```python
from build123d import *

# Parameters (mm, degrees)
F0_R          = 54.61
F0_R_2        = 51.435
F1_DEPTH      = 3.175
F2_R          = 1.27
F3_DEPTH      = 59.69
F3_DEPTH_BACK = 59.69
F4_R          = 51.435
F5_DEPTH      = 25.4
F6_R          = 1.524
F7_DEPTH      = 53.975
F7_DEPTH_BACK = 53.975


with BuildPart() as f1:
    # F0 (on Top) → F1 (new body)
    with BuildSketch(Plane.XY):
        Circle(F0_R)
        Circle(F0_R_2, mode=Mode.SUBTRACT)
    extrude(amount=F1_DEPTH)

    # F2 (on Front) → F3 (join, two sides)
    with BuildSketch(Plane.XZ) as f3_sk:
        with Locations((0, 1.5875)):
            Circle(F2_R)
    extrude(amount=F3_DEPTH)
    extrude(f3_sk.sketch, amount=-F3_DEPTH_BACK)

    # F4 (on Top) → F5 (cut)
    with BuildSketch(Plane.XY):
        Circle(F4_R)
    extrude(amount=F5_DEPTH, mode=Mode.SUBTRACT)

    # F6 (on Right) → F7 (cut, two sides)
    with BuildSketch(Plane.YZ) as f7_sk:
        with Locations((0, 1.5875)):
            Circle(F6_R)
    extrude(amount=-F7_DEPTH, mode=Mode.SUBTRACT)
    extrude(f7_sk.sketch, amount=F7_DEPTH_BACK, mode=Mode.SUBTRACT)


solid = f1.part
```
Geometry check sheet. Reference: the model listing, model coordinates, mm. A direction names the side the tool comes from. Give positions to 0.01 mm unless a question says otherwise; leave off trailing zeros. Write each loop counter-clockwise with the first axis right and the second up, starting at its lowest first coordinate (ties: lowest second). Pieces come first, ordered by that corner, then holes. Notation, with made-up numbers: (31, -30.5) - (55, -30.5) arc R21 cw to (55, -26.5) - close; hole circle Ø9 at (53, -19.5). An arc over 180 degrees is marked (long way). Use a Markdown table: item, result.
Q1. Set-up check for faces 4 (the face through (0, 59.69, 2)), 5 (the face through (-0.28, -57.11, 0.35)), 6 (the face through (-37, -36, 0)), 7 (the face through (-52.676, 0.703, 0.235)), 8 (the face through (-0.28, 57.11, 0.35)): record each of +Z, -Z, +X, -X, +Y, -Y from which the full face is reachable in a straight line by a thin tool's end or side.
Computed:
| item | result |
|---|---|
| face 4 | +Z, -Z, +X, -X, +Y |
| face 5 | -Y |
| face 6 | -Z, +X, -X, +Y, -Y |
| face 7 | none |
| face 8 | +Y |
Q2. Go/stop test with flat-tipped pins: P1, Ø1.5, axis at x = 19, z = 2, coming from the -Y side; P2, Ø1.5, axis at y = -15, z = 2, coming from the -X side. Record where each tip stops, or that it passes through.
Computed:
| item | result |
|---|---|
| P1 | stops at y = -51.47 |
| P2 | stops at x = -52.72 |
Q3. Thickness scan on L1, parallel to Y at x = 0, z = 2.05 (3 decimals); L2, parallel to Y at x = -9, z = 1; L3, parallel to X at y = 13.5, z = 2.2. Record the ranges inside material, lowest first. Write a range as [from, to].
Computed:
| item | result |
|---|---|
| L1 | y = [-59.69, -51.435], [51.435, 59.69] |
| L2 | y = [-53.86, -50.64], [50.64, 53.86] |
| L3 | x = [-52.92, -49.63], [49.63, 52.92] |
Q4. Draft check along Z on faces 1 (the face through (0, -59.69, 2)), 2 (the face through (-37, -36, 3.175)), 3 (the face through (-53.975, 0, 2)). Enter one of: pulls with the +Z half, pulls with the -Z half, needs draft (parallel to the pull), parting line crosses it, or undercut.
Computed:
| item | result |
|---|---|
| face 1 | needs draft |
| face 2 | pulls with the +Z half |
| face 3 | undercut |
Q5. Section check D-D, the plane y = 45. Enter the section's corners in (x, z) (1 decimal).
Computed:
| item | result |
|---|---|
| outline | (-30.9, 0) - (-24.9, 0) - (-24.9, 3.2) - (-30.9, 3.2) - close; (24.9, 0) - (30.9, 0) - (30.9, 3.2) - (24.9, 3.2) - close |
Q6. Section check C-C, the plane z = 2.1. Enter the section's corners in (x, y) (3 decimals).
Computed:
| item | result |
|---|---|
| outline | (-1.162, -59.69) - (1.162, -59.69) - (1.162, -54.598) arc R54.61 ccw to (1.162, 54.598) - (1.162, 59.69) - (-1.162, 59.69) - (-1.162, 54.598) arc R54.61 ccw to (-1.162, -54.598) - close; hole (-53.975, -1.435) - (-51.415, -1.435) arc R51.435 ccw to (51.415, -1.435) - (53.975, -1.435) - (53.975, 1.435) - (51.415, 1.435) arc R51.435 ccw to (-51.415, 1.435) - (-53.975, 1.435) - close |
Q7. Section check B-B, the plane x = 46. Enter the section's corners in (y, z) (3 decimals).
Computed:
| item | result |
|---|---|
| outline | (-29.432, 0) - (-23.012, 0) - (-23.012, 3.175) - (-29.432, 3.175) - close; (23.012, 0) - (29.432, 0) - (29.432, 3.175) - (23.012, 3.175) - close |
